Source: CAD feature listing. Evaluate the final solid. Frame: model axes, mm. A direction names the side the tool comes from. Give positions to 0.01 mm unless a question says otherwise; leave off trailing zeros. Order: outer loops, then holes, each group sorted by start corner. A loop starts at its lowest first (then second) coordinate and runs counter-clockwise, first axis right, second up.
from build123d import *

# Parameters (mm, degrees)
SKETCH1_R           = 6.375
BOSS_EXTRUDE1_DEPTH = 15
SKETCH9_R           = 10
BOSS_EXTRUDE5_DEPTH = 15
SKETCH10_R          = 7.75
CUT_EXTRUDE4_DEPTH  = 10
SKETCH11_R          = 7.75
CUT_EXTRUDE5_DEPTH  = 7
CUT_EXTRUDE5_DRAFT  = -35
SKETCH12_R          = 4.125
CUT_EXTRUDE6_DEPTH  = 20
CHAMFER1_SIZE       = 4
CHAMFER1_SIZE2      = 0.420416941
CHAMFER2_SIZE       = 4
CHAMFER2_SIZE2      = 0.420416941
FILLET2_R           = 2


with BuildPart() as part:
    # Sketch1 → Boss-Extrude1 (new body)
    with BuildSketch(Plane(origin=(0, 0, 0), x_dir=(1, 0, 0), z_dir=(0, 1, 0))):
        with Locations(Location((0, 0, 0), (0, 0, 270))):
            Circle(SKETCH1_R)
    extrude(amount=BOSS_EXTRUDE1_DEPTH)

    # Sketch9 → Boss-Extrude5 (add)
    with BuildSketch(Plane(origin=(0, 15, 0), x_dir=(1, 0, 0), z_dir=(0, 1, 0))):
        with Locations(Location((0, 0, 0), (0, 0, 270))):
            Circle(SKETCH9_R)
    extrude(amount=BOSS_EXTRUDE5_DEPTH)

    # Sketch10 → Cut-Extrude4 (cut)
    with BuildSketch(Plane(origin=(0, 30, 0), x_dir=(1, 0, 0), z_dir=(0, 1, 0))):
        with Locations(Location((0, 0, 0), (0, 0, 270))):
            Circle(SKETCH10_R)
    extrude(amount=-CUT_EXTRUDE4_DEPTH, mode=Mode.SUBTRACT)


with BuildPart() as cut_extrude5_tool:
    # Sketch11 → Cut-Extrude5 (with draft: the straight prism first)
    with BuildSketch(Plane(origin=(0, 20, 0), x_dir=(1, 0, 0), z_dir=(0, 1, 0))):
        with Locations(Location((0, 0, 0), (0, 0, 270))):
            Circle(SKETCH11_R)
    extrude(amount=-CUT_EXTRUDE5_DEPTH)
    # Cut-Extrude5: the draft: its side faces are tilted about the plane it starts from
    cut_extrude5_sides = [cut_extrude5_tool.faces().sort_by_distance(p)[0] for p in [
        (0, 16.5, -7.75),
    ]]
    draft(cut_extrude5_sides, Plane(origin=(0, 20, 0), x_dir=(1, 0, 0), z_dir=(0, 1, 0)), CUT_EXTRUDE5_DRAFT)


with BuildPart() as part_1:
    add(part.part)

    # Cut-Extrude5: cut by cut_extrude5_tool
    add(cut_extrude5_tool.part, mode=Mode.SUBTRACT)

    # Sketch12 → Cut-Extrude6 (cut)
    with BuildSketch(Plane.XZ):
        with Locations(Location((0, 0, 0), (0, 0, 270))):
            Circle(SKETCH12_R)
    extrude(amount=-CUT_EXTRUDE6_DEPTH, mode=Mode.SUBTRACT)

    # Chamfer1
    chamfer1_edges = [part_1.edges().sort_by_distance(p)[0] for p in [
        (0, 30, -10),
    ]]
    chamfer1_side = [part_1.faces().sort_by_distance(p)[0] for p in [
        (0, 22.5, -10),
    ]]
    chamfer(chamfer1_edges, length=CHAMFER1_SIZE, length2=CHAMFER1_SIZE2, reference=chamfer1_side[0])

    # Chamfer2
    chamfer2_edges = [part_1.edges().sort_by_distance(p)[0] for p in [
        (0, 0, -6.375),
    ]]
    chamfer2_side = [part_1.faces().sort_by_distance(p)[0] for p in [
        (0, 7.5, -6.375),
    ]]
    chamfer(chamfer2_edges, length=CHAMFER2_SIZE, length2=CHAMFER2_SIZE2, reference=chamfer2_side[0])

    # Fillet2
    fillet2_edges = [part_1.edges().sort_by_distance(p)[0] for p in [
        (0, 15, -10),
    ]]
    fillet(fillet2_edges, radius=FILLET2_R)


solid = part_1.part
(1) Section A-A, the plane z = 0. Return loops of the section in (x, y) (3 decimals).
(2) Pin query (flat end, axial travel): pin 1 Ø10 at (x, z) = (6.5, -4) entering from +Y; pin 2 Ø1 at (x, y) = (6.5, 15) entering from +Z; pin 3 Ø12 at (x, y) = (7.5, 7.5) entering from +Z. Return the tip coordinate at first contact, or that it passes through.
(3) Section C-C, the plane y = 10. Return loops of the section in (x, z) (3 decimals).
(4) Line query: line 1 along X through (y, z) = (24.5, 0); line 2 along X through (y, z) = (6.5, 0) (3 decimals); line 3 along Y through (x, z) = (5.25, -5.75). Output: solid intervals per line, ascending.
(5) Section D-D, the plane y = 25. Return loops of the section in (x, z), plus the area to 3 significant figures.
(6) Section B-B, the plane x = 0. Return loops of the section in (y, z) (3 decimals), plus the area to 3 significant figures.
(7) Access query for faces 1 (the flat face through (-6.5, 15, -0.6)), 2 (the flat face through (0, 30, 8)). Directions: +Z, -Z, +X, -X, +Y, -Y. A direction counts if a zero-diameter tool reaches every point of the face in a straight line with its end or side. Return the directions, or none.
(8) Draft query along X for faces 3 (the flat face through (4.1, 0, -1.4)), 4 (the cylindrical face through (-6.223, 9.423, -1.382)), 5 (the cylindrical face through (7.684, 25.07, -1.009)). Return one class per face: +X half, -X half, draft (parallel to the pull), parting line (faces both ways), or undercut.
Checks:
1. outline: (-10, 17) arc R2 ccw to (-8, 15) - (-6.375, 15) - (-6.375, 4) - (-5.955, 0) - (-4.125, 0) - (-4.125, 14.823) - (-7.75, 20) - (-7.75, 30) - (-9.58, 30) - (-10, 26) - close; (4.125, 0) - (5.955, 0) - (6.375, 4) - (6.375, 15) - (8, 15) arc R2 ccw to (10, 17) - (10, 26) - (9.58, 30) - (7.75, 30) - (7.75, 20) - (4.125, 14.823) - close
2. pin 1: stops at y = 30
2. pin 2: stops at z = 6.81
2. pin 3: stops at z = 6.2
3. outline: circle Ø12.75 at (0, 0); hole circle Ø8.25 at (0, 0)
4. line 1: x = -10 to -7.75, 7.75 to 10
4. line 2: x = -6.375 to -4.125, 4.125 to 6.375
4. line 3: y = 15 to 30
5. outline: circle Ø20 at (0, 0); hole circle Ø15.5 at (0, 0)
5. area: 125 mm2
6. outline: (0, -5.955) - (4, -6.375) - (15, -6.375) - (15, -8) arc R2 ccw to (17, -10) - (26, -10) - (30, -9.58) - (30, -7.75) - (20, -7.75) - (14.823, -4.125) - (0, -4.125) - close; (0, 4.125) - (14.823, 4.125) - (20, 7.75) - (30, 7.75) - (30, 9.58) - (26, 10) - (17, 10) arc R2 ccw to (15, 8) - (15, 6.375) - (4, 6.375) - (0, 5.955) - close
6. area: 147 mm2
7. face 1: -Y
7. face 2: +Z, -Z, +X, -X, +Y
8. face 3: draft
8. face 4: parting line
8. face 5: undercut
